Autodesk Inventor part; units mm, degrees
ref_plane "YZ Plane" through (0, 0, 0) normal (1, 0, 0) x (0, 1, 0)
ref_plane "XZ Plane" through (0, 0, 0) normal (0, 1, 0) x (-1, 0, 0)
ref_plane "XY Plane" through (0, 0, 0) normal (0, 0, 1) x (1, 0, 0)
sketch "Sketch1" plane through (0, 0, 0) normal (0, 0, 1) x (1, 0, 0)
  circle A0 centre (0, 0) radius 4.62
  circle A1 centre (0, 0) radius 5
  dimension "d0" = 9.24
  dimension "d1" = 10
extrude "Extrusion1" add sketch "Sketch1" along normal blind 180
sketch "Sketch7" plane through (0, 0, 0) normal (0, 0, -1) x (-1, 0, 0)
  circle A0 centre (0, 0) radius 4
extrude "Extrusion6" add sketch "Sketch7" against normal blind 10
sketch "Sketch8" plane through (0, 0, 0) normal (0, 0, -1) x (-1, 0, 0)
  circle A0 centre (0, 0) radius 4.8
  dimension "d23" = 9.6
extrude "Extrusion7" add sketch "Sketch8" along normal blind 6
chamfer "Chamfer1" distance 1.5 angle 45 1 edges at (4.8, 0, -6)
properties part number "Acrylic 8 ID, 10 OD" material "Glass"
Geometry check sheet. Reference: the model listing, model coordinates, mm. A direction names the side the tool comes from. Round coordinates to 2 decimals unless told otherwise and drop trailing zeros. Order: outer loops, then holes, each group sorted by start corner. A loop starts at its lowest first (then second) coordinate and runs counter-clockwise, first axis right, second up. Notation, with made-up numbers: M 75,-1.5 L 128,-1.5 A23 ccw 128,14.5 Z; hole C 79.25,81.25 d3. An arc over 180 degrees is marked long. Answer in a Markdown table with one row per item.
(1) Tool access check on faces 1 (the face through (-2.58, -4.05, -2.22)), 2 (the face through (0.867, -3.905, 4.93)). Record the directions out of +Z, -Z, +X, -X, +Y, -Y that give a thin tool (end or side, any length) a straight path to the whole face; none if there is none.
Responses:
| item | result |
|---|---|
| face 1 | -Z |
| face 2 | +Z |
(2) Scan lines: probe 1 along Y at (x, z) = (0, 112); probe 2 along Z at (x, y) = (-4, 1.5); probe 3 along Y at (x, z) = (3, 41.5). Record each from-to range of solid material in increasing order. Write a range as from..to.
Responses:
| item | result |
|---|---|
| probe 1 | y = -5..-4.62, 4.62..5 |
| probe 2 | z = -5.03..0 |
| probe 3 | y = -4..-3.51, 3.51..4 |
(3) Draft check along X on faces 3 (the face through (1.7, 3.8, 0)), 4 (the face through (-1.08, 4.88, 88.74)), 5 (the face through (0, 0, -6)), 6 (the face through (0, 0, 10)). Enter one of: released by +X, released by -X, zero draft, split by the parting line, or undercut.
Responses:
| item | result |
|---|---|
| face 3 | undercut |
| face 4 | split by the parting line |
| face 5 | zero draft |
| face 6 | undercut |
(4) Go/stop test with flat-tipped pins: P1, Ø2, axis at x = -2.5, z = 108.5, coming from the +Y side; P2, Ø1.5, axis at x = 1.5, z = 79, coming from the +Y side; P3, Ø1.5, axis at x = -1, y = 0, coming from the +Z side. Record where each tip stops, or that it passes through.
Responses:
| item | result |
|---|---|
| P1 | stops at y = 4.77 |
| P2 | stops at y = 4.94 |
| P3 | stops at z = 10 |
(5) Sectioned sample at C-C, the plane z = 162. Record the cut outline in (x, y).
Responses:
| item | result |
|---|---|
| outline | C 0,0 d10; hole C 0,0 d9.24 |
(6) Sectioned sample at A-A, the plane y = 0. Record the cut outline in (x, z), and give its area (3 significant figures).
Responses:
| item | result |
|---|---|
| outline | M -5,0 L -4.8,0 L -4.8,-4.5 L -3.3,-6 L 3.3,-6 L 4.8,-4.5 L 4.8,0 L 5,0 L 5,180 L 4.62,180 L 4.62,0 L 4,0 L 4,10 L -4,10 L -4,0 L -4.62,0 L -4.62,180 L -5,180 Z |
| area | 272 mm² |
